The model under review builds one solid part; all positions refer to its coordinate system, in mm. A direction names the side the tool comes from. Give positions to 0.01 mm unless a question says otherwise; leave off trailing zeros. Write each loop counter-clockwise with the first axis right and the second up, starting at its lowest first coordinate (ties: lowest second). Pieces come first, ordered by that corner, then holes.
from build123d import *

# Parameters (mm, degrees)
F0_W     = 67.1
F0_H     = 138.3
F1_DEPTH = 3.55
F2_R     = 10
F3_T     = -2.5
F4_R     = 5.246846
F5_DEPTH = 12.5
F6_W     = 33.990787
F6_H     = 7.1
F7_DEPTH = 3
F8_R     = 2.352269
F9_DEPTH = 12.5


with BuildPart() as f1:
    # F0 (on Front) → F1 (new body, symmetric)
    with BuildSketch(Plane.XZ):
        Rectangle(F0_W, F0_H)
    extrude(amount=F1_DEPTH, both=True)

    # F2
    f2_edges = [f1.edges().sort_by_distance(p)[0] for p in [
        (33.55, 0, -69.15),
        (33.55, 0, 69.15),
        (-33.55, 0, -69.15),
        (-33.55, 0, 69.15),
    ]]
    fillet(f2_edges, radius=F2_R)

    # F3
    f3_openings = [f1.faces().sort_by_distance(p)[0] for p in [
        (0, -3.55, 0),
    ]]
    offset(amount=F3_T, openings=f3_openings)

    # F4 (on Front) → F5 (cut, symmetric)
    with BuildSketch(Plane.XZ):
        with Locations((16.993571, 58.656055)):
            Circle(F4_R)
    extrude(amount=F5_DEPTH, both=True, mode=Mode.SUBTRACT)

    # F6 (on face) → F7 (cut, symmetric)
    with BuildSketch(Plane(origin=(0, 0, -69.15), x_dir=(1, 0, 0), z_dir=(0, 0, -1))):
        with Locations((0.352152, 0)):
            Rectangle(F6_W, F6_H)
    extrude(amount=F7_DEPTH, both=True, mode=Mode.SUBTRACT)

    # F8 (on Front) → F9 (cut, symmetric)
    with BuildSketch(Plane.XZ):
        with Locations((6.732481, 61.507728)):
            Circle(F8_R)
    extrude(amount=F9_DEPTH, both=True, mode=Mode.SUBTRACT)


solid = f1.part
1) Consider section B-B, the plane y = -1.25. Give the boundary of the cut face in (x, z), then the cut area to 3 significant figures.
2) Insertion check: pin 1 (3.5 mm diameter, centred on x = 8, y = -2, fed in from -Z); pin 2 (1 mm diameter, centred on x = -22, z = 47, fed in from -Y); pin 3 (9.5 mm diameter, centred on x = 16.99, z = 58.66, fed in from +Y); pin 4 (1 mm diameter, centred on x = -8.5, y = 1.5, fed in from -Z). Each pin has a flat end and moves straight along its axis. Give the tip position at first contact, or say it passes through.
3) Consider section A-A, the plane x = 16. Give the boundary of the cut face in (y, z), then the cut area to 3 significant figures.
4) Consider section D-D, the plane z = 55.5. Give the boundary of the cut face in (x, y), then the cut area to 3 significant figures.
5) Consider section C-C, the plane z = 37.5. Give the boundary of the cut face in (x, y), then the cut area to 3 significant figures.
6) To check wall thickness, follow probe 1 along X at (y, z) = (-2, 11.5); probe 2 along Y at (x, z) = (28, 31.5); probe 3 along Z at (x, y) = (-9, -0.25). State the ranges of each line that lie inside material, in increasing order.
7) Tool access review of faces 1 (the cylindrical face through (-28.911, -1.282, -64.395)), 2 (the flat face through (-20, 0, -69.15)), 3 (the flat face through (0, 2, -66.15)): name each direction out of +Z, -Z, +X, -X, +Y, -Y from which nothing blocks a thin tool from reaching the whole face with its end or side.
8) The part is to be moulded in two halves that separate along Z. For faces 4 (the flat face through (0, 0, 69.15)), 5 (the flat face through (32, -3.55, 16)), 6 (the flat face through (20, 0, -69.15)), 7 (the cylindrical face through (28.911, -1.218, 64.395)), say which applies: +Z half, -Z half, draft (parallel to the pull), parting line (faces both ways), or undercut.
Answer block:
1. outline: (-33.55, -59.15) arc R10 ccw to (-23.55, -69.15) - (-16.64, -69.15) - (-16.64, -66.65) - (-23.55, -66.65) arc R7.5 cw to (-31.05, -59.15) - (-31.05, 59.15) arc R7.5 cw to (-23.55, 66.65) - (23.55, 66.65) arc R7.5 cw to (31.05, 59.15) - (31.05, -59.15) arc R7.5 cw to (23.55, -66.65) - (17.35, -66.65) - (17.35, -69.15) - (23.55, -69.15) arc R10 ccw to (33.55, -59.15) - (33.55, 59.15) arc R10 ccw to (23.55, 69.15) - (-23.55, 69.15) arc R10 ccw to (-33.55, 59.15) - close
1. area: 879 mm2
2. pin 1: stops at z = 66.65
2. pin 2: stops at y = 1.05
2. pin 3: passes through
2. pin 4: stops at z = -66.15
3. outline: (-3.55, 66.65) - (1.05, 66.65) - (1.05, 63.81) - (3.55, 63.81) - (3.55, 69.15) - (-3.55, 69.15) - close; (1.05, -66.15) - (3.55, -66.15) - (3.55, 53.5) - (1.05, 53.5) - close
3. area: 324 mm2
4. outline: (-33.55, -3.55) - (-31.05, -3.55) - (-31.05, 1.05) - (12.8, 1.05) - (12.8, 3.55) - (-33.55, 3.55) - close; (21.19, 1.05) - (31.05, 1.05) - (31.05, -3.55) - (33.55, -3.55) - (33.55, 3.55) - (21.19, 3.55) - close
4. area: 170 mm2
5. outline: (-33.55, -3.55) - (-31.05, -3.55) - (-31.05, 1.05) - (31.05, 1.05) - (31.05, -3.55) - (33.55, -3.55) - (33.55, 3.55) - (-33.55, 3.55) - close
5. area: 191 mm2
6. probe 1: x = -33.55 to -31.05, 31.05 to 33.55
6. probe 2: y = 1.05 to 3.55
6. probe 3: z = 66.65 to 69.15
7. face 1: -Y
7. face 2: -Z, +X, -X, +Y, -Y
7. face 3: -Z, +Y, -Y
8. face 4: +Z half
8. face 5: draft
8. face 6: -Z half
8. face 7: undercut
